Could you check a few things on this drawing? It's one solid part, dimensions in mm from its lowest x, y, z. Coordinates: 2 decimals unless noted, no trailing zeros. Order: outer loops, then holes, each group sorted by start corner. A loop starts at its lowest first (then second) coordinate and runs counter-clockwise, first axis right, second up. Notation, with made-up numbers: (37, 86.25) - (51, 86.25) arc R21 ccw to (51, 108.25) - close; hole circle Ø1 at (12.5, 47.25). An arc over 180 degrees is marked (long way). Return JSON: item names as keys, results as strings. Group by question number.
1) Imagine slicing it at D-D (z = 2). Write out the boundary of the cut face in (x, y), and give its area (3 significant figures).
2) If I drill on line 1 along Y through (x, z) = (6.5, 0.7); line 2 along Z through (x, y) = (7.25, 5.75); line 3 along X through (y, z) = (18, 2.55), over which ranges is the centre line in solid material (lowest first)?
3) Imagine slicing it at A-A (x = 6). Write out the boundary of the cut face in (y, z), and give its area (3 significant figures).
4) Imagine slicing it at C-C (z = 0.8). Write out the boundary of the cut face in (x, y).
5) For pin 1 Ø1.1 at (x, z) = (7, 2.5) entering from +Y; pin 2 Ø1.8 at (x, y) = (6.5, 3) entering from +Z; pin 3 Ø0.5 at (y, z) = (18.5, 2) entering from -X; pin 4 Ø1.5 at (x, y) = (3, 11) entering from +Z, each with a flat end and sliding along its axis, tell me the tip position at first contact or that it passes through.
6) If we mould it in two halves opening along X, with no side actions, what happens to the marked faces 1, 2, 3 and 4? For each: pulls with the +X half, pulls with the -X half, needs draft (parallel to the pull), parting line crosses it, or undercut.
7) Imagine slicing it at B-B (y = 3). Write out the boundary of the cut face in (x, z), and give its area (3 significant figures).
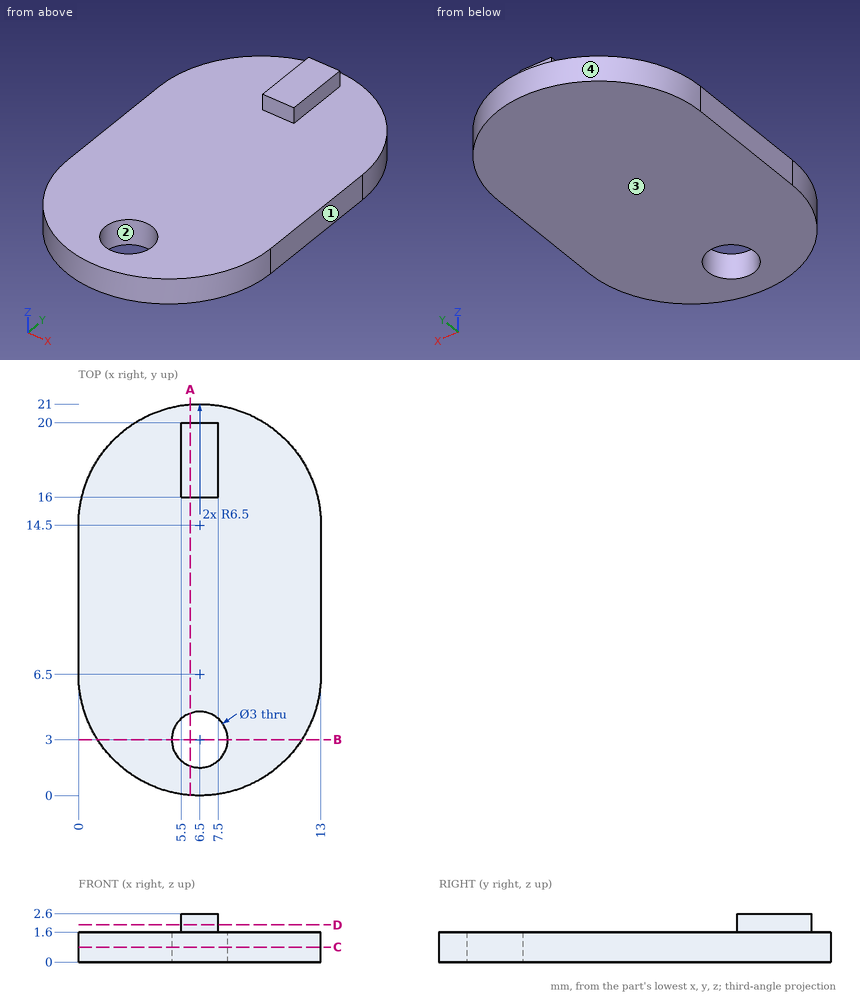
Calculated:
{
 "1": {"outline": "(5.5, 16) - (7.5, 16) - (7.5, 20) - (5.5, 20) - close", "area": "8.00 mm2"},
 "2": {"line 1": "0 to 1.5, 4.5 to 21", "line 2": "0 to 1.6", "line 3": "5.5 to 7.5"},
 "3": {"outline": "(0.02, 0) - (1.59, 0) - (1.59, 1.6) - (0.02, 1.6) - close; (4.41, 0) - (20.98, 0) - (20.98, 1.6) - (20, 1.6) - (20, 2.6) - (16, 2.6) - (16, 1.6) - (4.41, 1.6) - close", "area": "33.0 mm2"},
 "4": {"outline": "(0, 6.5) arc R6.5 ccw to (13, 6.5) - (13, 14.5) arc R6.5 ccw to (0, 14.5) - close; hole circle Ø3 at (6.5, 3)"},
 "5": {"pin 1": "y = 20", "pin 2": "through", "pin 3": "x = 5.5", "pin 4": "z = 1.6"},
 "6": {"face 1": "pulls with the +X half", "face 2": "undercut", "face 3": "needs draft", "face 4": "parting line crosses it"},
 "7": {"outline": "(1.02, 0) - (5, 0) - (5, 1.6) - (1.02, 1.6) - close; (8, 0) - (11.98, 0) - (11.98, 1.6) - (8, 1.6) - close", "area": "12.7 mm2"}
}
